Geometry: final body of the model. Coordinates: model frame, mm. Face numbers are marked on the shaded views. Give positions to 0.01 mm unless a question says otherwise; leave off trailing zeros. Order: outer loops, then holes, each group sorted by start corner. A loop starts at its lowest first (then second) coordinate and runs counter-clockwise, first axis right, second up. Notation, with made-up numbers: (7.5, 74) - (35.5, 74) arc R9 ccw to (35.5, 84) - close; hole circle Ø7 at (52.25, 58). An arc over 180 degrees is marked (long way). One line per question, with ' | ' between items. Start each with the question number.
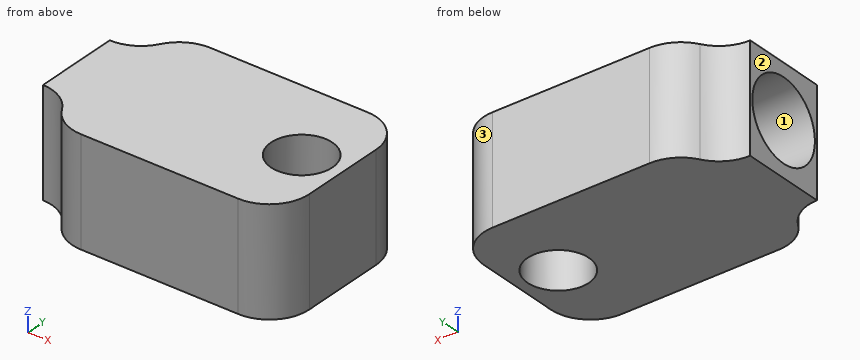
from build123d import *

# Parameters (mm, degrees)
F0_R     = 1.15
F1_DEPTH = 4
F2_R     = 1.5
F3_R     = 1.5
F4_DEPTH = 4


with BuildPart() as f1:
    # F0 (on Top) → F1 (new body)
    with BuildSketch(Plane.XY):
        with BuildLine():
            Line((3.5, 3.1), (-3.5, 3.1))
            ThreePointArc((-3.5, 3.1), (-3.93934, 2.03934), (-5, 1.6))
            Line((-5, 1.6), (-5, -1.6))
            ThreePointArc((-5, -1.6), (-3.93934, -2.03934), (-3.5, -3.1))
            Line((-3.5, -3.1), (3.5, -3.1))
            ThreePointArc((3.5, -3.1), (4.56066, -2.66066), (5, -1.6))
            Line((5, -1.6), (5, 1.6))
            ThreePointArc((5, 1.6), (4.56066, 2.66066), (3.5, 3.1))
        make_face()
        with Locations((3.457711, 0)):
            Circle(F0_R, mode=Mode.SUBTRACT)
    extrude(amount=F1_DEPTH)

    # F2
    f2_edges = [f1.edges().sort_by_distance(p)[0] for p in [
        (-3.5, -3.1, 2),
        (-3.5, 3.1, 2),
    ]]
    fillet(f2_edges, radius=F2_R)

    # F3 (on face) → F4 (cut)
    with BuildSketch(Plane(origin=(-5, 0, 0), x_dir=(0, -1, 0), z_dir=(-1, 0, 0))):
        with Locations((0, 2)):
            Circle(F3_R)
    extrude(amount=-F4_DEPTH, mode=Mode.SUBTRACT)


solid = f1.part
(1) Pull-direction query (Y, two-part tool) for the marked faces 1, 2 and 3; classes: +Y half, -Y half, draft (parallel to the pull), parting line (faces both ways), or undercut.
(2) Cut plane B-B, the plane z = 2. Return the cut outline in (x, y), plus the area to 3 significant figures.
(3) Cut plane A-A, the plane y = 0. Return the cut outline in (x, z).
(4) Material intervals for line 1 along Z through (x, y) = (-2.5, 1.25); line 2 along X through (y, z) = (-1, 3.2); line 3 along X through (y, z) = (0.75, 3.1), sorted ascending. Write a range as from..to.
(5) Cut plane D-D, the plane y = 0.75. Return the cut outline in (x, z), plus the area to 3 significant figures.
(6) Contact query for flat-ended pins moving along their axis: P1, Ø0.9, axis at y = 0, z = 2, coming from the -X side; P2, Ø2.5, axis at x = 3.46, y = 0, coming from the -Z side. Output: stop coordinate, or through.
(7) Cut plane C-C, the plane z = 0.7. Return the cut outline in (x, y), plus the area to 3 significant figures.
Results are:
1) face 1: undercut | face 2: draft | face 3: +Y half
2) outline: (-5, -1.6) arc R1.5 cw to (-3.7, -2.35) arc R1.5 ccw to (-2.4, -3.1) - (3.5, -3.1) arc R1.5 ccw to (5, -1.6) - (5, 1.6) arc R1.5 ccw to (3.5, 3.1) - (-2.4, 3.1) arc R1.5 ccw to (-3.7, 2.35) arc R1.5 cw to (-5, 1.6) - (-5, 1.5) - (-1, 1.5) - (-1, -1.5) - (-5, -1.5) - close; hole circle Ø2.3 at (3.46, 0) | area: 41.0 mm2
3) outline: (-5, 0) - (2.31, 0) - (2.31, 4) - (-5, 4) - (-5, 3.5) - (-1, 3.5) - (-1, 0.5) - (-5, 0.5) - close; (4.61, 0) - (5, 0) - (5, 4) - (4.61, 4) - close
4) line 1: 0..1.17, 2.83..4 | line 2: -5..2.89, 4.03..5 | line 3: -1..2.59, 4.33..5
5) outline: (-5, 0) - (2.59, 0) - (2.59, 4) - (-5, 4) - (-5, 3.3) - (-1, 3.3) - (-1, 0.7) - (-5, 0.7) - close; (4.33, 0) - (5, 0) - (5, 4) - (4.33, 4) - close | area: 22.6 mm2
6) P1: x = -1 | P2: z = 0
7) outline: (-5, -1.6) arc R1.5 cw to (-3.7, -2.35) arc R1.5 ccw to (-2.4, -3.1) - (3.5, -3.1) arc R1.5 ccw to (5, -1.6) - (5, 1.6) arc R1.5 ccw to (3.5, 3.1) - (-2.4, 3.1) arc R1.5 ccw to (-3.7, 2.35) arc R1.5 cw to (-5, 1.6) - (-5, 0.75) - (-1, 0.75) - (-1, -0.75) - (-5, -0.75) - close; hole circle Ø2.3 at (3.46, 0) | area: 47.0 mm2
